from build123d import *

# Parameters (mm, degrees)
BASE_FLANGE1_DEPTH    = 2
F_5_0MM_DOWEL_HOLE1_D = 7
F_5_0MM_DOWEL_HOLE2_D = 5


# Sheet-metal steps are written as plain solids
with BuildPart() as part:
    # Sketch1 → Base-Flange1 (new body)
    with BuildSketch(Plane(origin=(0, 0, 0), x_dir=(1, 0, 0), z_dir=(0, 1, 0))):
        with BuildLine():
            Line((92, -12.5), (-92, -12.5))
            ThreePointArc((-92, -12.5), (-94.121320344, -11.621320344), (-95, -9.5))
            Line((-95, -9.5), (-95, 9.5))
            ThreePointArc((-95, 9.5), (-94.121320344, 11.621320344), (-92, 12.5))
            Line((-92, 12.5), (92, 12.5))
            ThreePointArc((92, 12.5), (94.121320344, 11.621320344), (95, 9.5))
            Line((95, 9.5), (95, -9.5))
            ThreePointArc((95, -9.5), (94.121320344, -11.621320344), (92, -12.5))
        make_face()
    extrude(amount=BASE_FLANGE1_DEPTH)

    # Ø5.0mm Dowel Hole1 (through all)
    with Locations(Plane(origin=(0, 2, 0), x_dir=(1, 0, 0), z_dir=(0, 1, 0))):
        with Locations((-80, 0), (80, 0)):
            Hole(F_5_0MM_DOWEL_HOLE1_D / 2)

    # Ø5.0mm Dowel Hole2 (through all)
    with Locations(Plane(origin=(0, 2, 0), x_dir=(1, 0, 0), z_dir=(0, 1, 0))):
        with Locations((-60, 0), (-40, 0)):
            Hole(F_5_0MM_DOWEL_HOLE2_D / 2)


solid = part.part
Geometry: final body of the model. Coordinates: model frame, mm. Coordinates: 2 decimals unless noted, no trailing zeros. Loops run counter-clockwise (first coordinate to the right, second up) from the corner with the lowest first, then second, coordinate; pieces in that order, holes last. Notation, with made-up numbers: M 74,73.25 L 115,73.25 A20 cw 115,89.25 Z; hole C 72.5,27.25 d9. An arc over 180 degrees is marked long. One line per item, written item: value. Start each with the question number.
1) Cut plane A-A (z = 0). Return loops of the section in (x, y).
2) Cut plane C-C (x = -80). Return loops of the section in (y, z).
3) Pin query (flat end, axial travel): P1, Ø4.5, axis at x = -40, z = 0, coming from the -Y side. Return the tip coordinate at first contact, or that it passes through.
4) Cut plane B-B (y = 0.75). Return loops of the section in (x, z), then the cut area to 3 significant figures.
5) Draft query along X for faces 1 (the cylindrical face through (-94.1, 0.99, 11.64)), 2 (the cylindrical face through (-83.233, 0.986, 1.341)), 3 (the flat face through (1, 0, 0)). Return one class per face: released by +X, released by -X, zero draft, split by the parting line, or undercut.
6) Cut plane D-D (x = -40). Return loops of the section in (y, z), then the cut area to 3 significant figures.
7) Material intervals for L1, parallel to X at y = 1.4, z = -3; L2, parallel to Z at x = 80, y = 1.05; L3, parallel to Z at x = -60, y = 1.45, sorted ascending. Write a range as from..to.
Evaluation:
1. outline: M -95,0 L -83.5,0 L -83.5,2 L -95,2 Z; M -76.5,0 L -62.5,0 L -62.5,2 L -76.5,2 Z; M -57.5,0 L -42.5,0 L -42.5,2 L -57.5,2 Z; M -37.5,0 L 76.5,0 L 76.5,2 L -37.5,2 Z; M 83.5,0 L 95,0 L 95,2 L 83.5,2 Z
2. outline: M 0,-12.5 L 2,-12.5 L 2,-3.5 L 0,-3.5 Z; M 0,3.5 L 2,3.5 L 2,12.5 L 0,12.5 Z
3. P1: through
4. outline: M -95,-9.5 A3 ccw -92,-12.5 L 92,-12.5 A3 ccw 95,-9.5 L 95,9.5 A3 ccw 92,12.5 L -92,12.5 A3 ccw -95,9.5 Z; hole C -80,0 d7; hole C -60,0 d5; hole C -40,0 d5; hole C 80,0 d7
4. area: 4,630 mm^2
5. face 1: released by -X
5. face 2: undercut
5. face 3: zero draft
6. outline: M 0,-12.5 L 2,-12.5 L 2,-2.5 L 0,-2.5 Z; M 0,2.5 L 2,2.5 L 2,12.5 L 0,12.5 Z
6. area: 40.0 mm^2
7. L1: -95..-81.8, -78.2..78.2, 81.8..95
7. L2: -12.5..-3.5, 3.5..12.5
7. L3: -12.5..-2.5, 2.5..12.5
